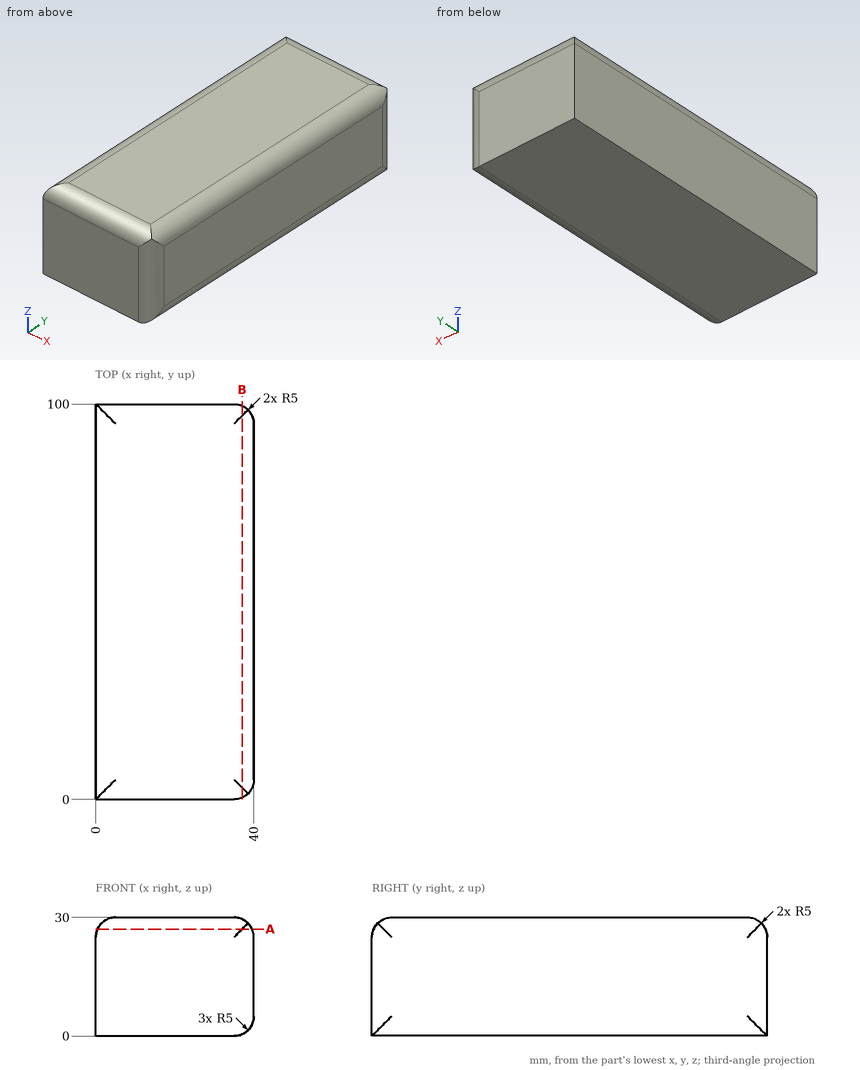
Could you check a few things on this drawing? It's one solid part, dimensions in mm from its lowest x, y, z. Give positions to 0.01 mm unless a question says otherwise; leave off trailing zeros. Write each loop counter-clockwise with the first axis right and the second up, starting at its lowest first coordinate (ties: lowest second). Pieces come first, ordered by that corner, then holes. Notation, with made-up numbers: (-17.5, 2.5) -> (20.5, 2.5) arc R20 ccw to (20.5, 41.5) -> close; hole circle Ø6 at (71, 82). An arc over 180 degrees is marked (long way). Write item = value, one per line.
(1) I need wall thicknesses on probe 1 along Y at (x, z) = (37.5, 18); probe 2 along X at (y, z) = (24, 28.5); probe 3 along X at (y, z) = (31, 4). Which ranges of each line are inside material? Lowest first, please. Write a range as from..to.
Worked out:
probe_1 = 0.67..99.33
probe_2 = 1.43..38.57
probe_3 = 0..39.9
(2) Suppose I cut it at A-A on z = 27. Write out the boundary of the cut face in (x, y), then the cut area to 3 significant figures.
Worked out:
outline = (0.42, 0.42) -> (37, 0.42) arc R5 ccw to (39.58, 3) -> (39.58, 97) arc R5 ccw to (37, 99.58) -> (0.42, 99.58) -> close
area = 3,880 mm^2
(3) Suppose I cut it at B-B on x = 37. Write out the boundary of the cut face in (y, z).
Worked out:
outline = (0.42, 0.42) -> (99.58, 0.42) -> (99.58, 27) arc R5 ccw to (97, 29.58) -> (3, 29.58) arc R5 ccw to (0.42, 27) -> close
